from build123d import *

# Parameters (mm, degrees)
SKETCH1_R           = 1.7
BOSS_EXTRUDE1_DEPTH = 13.5
CUT_EXTRUDE2_START  = -3.5
CUT_EXTRUDE2_DEPTH  = 3.5
BOSS_EXTRUDE2_DEPTH = 15.5
CHAMFER1_SIZE       = 3


with BuildPart() as part:
    # Sketch1 → Boss-Extrude1 (new body)
    with BuildSketch(Plane(origin=(0, 3, 0), x_dir=(1, 0, 0), z_dir=(0, 1, 0))):
        with BuildLine():
            Line((71.5, -48.5), (71.5, 48.5))
            ThreePointArc((71.5, 48.5), (70.621320344, 50.621320344), (68.5, 51.5))
            Line((68.5, 51.5), (-68.5, 51.5))
            ThreePointArc((-68.5, 51.5), (-70.621320344, 50.621320344), (-71.5, 48.5))
            Line((-71.5, 48.5), (-71.5, -48.5))
            ThreePointArc((-71.5, -48.5), (-70.621320344, -50.621320344), (-68.5, -51.5))
            Line((-68.5, -51.5), (68.5, -51.5))
            ThreePointArc((68.5, -51.5), (70.621320344, -50.621320344), (71.5, -48.5))
        make_face()
        with Locations(Location((-64, 44, 0), (0, 0, 90))):
            Circle(SKETCH1_R, mode=Mode.SUBTRACT)
        with Locations(Location((-64, -44, 0), (0, 0, 90))):
            Circle(SKETCH1_R, mode=Mode.SUBTRACT)
        with Locations(Location((64, -44, 0), (0, 0, 90))):
            Circle(SKETCH1_R, mode=Mode.SUBTRACT)
        with Locations(Location((64, 44, 0), (0, 0, 90))):
            Circle(SKETCH1_R, mode=Mode.SUBTRACT)
    extrude(amount=-BOSS_EXTRUDE1_DEPTH)

    # Sketch2 → Cut-Extrude2 (cut)
    with BuildSketch(Plane.XZ.offset(10.5).offset(CUT_EXTRUDE2_START)):
        with BuildLine():
            Line((-71.5, -40.5), (-63, -40.5))
            Line((-63, -40.5), (-60.5, -43))
            Line((-60.5, -43), (-60.5, -51.5))
            Line((-60.5, -51.5), (-68.5, -51.5))
            ThreePointArc((-68.5, -51.5), (-70.621320344, -50.621320344), (-71.5, -48.5))
            Line((-71.5, -48.5), (-71.5, -40.5))
        make_face()
        with BuildLine():
            Line((-71.5, 40.5), (-63, 40.5))
            Line((-63, 40.5), (-60.5, 43))
            Line((-60.5, 43), (-60.5, 51.5))
            Line((-60.5, 51.5), (-68.5, 51.5))
            ThreePointArc((-68.5, 51.5), (-70.621320344, 50.621320344), (-71.5, 48.5))
            Line((-71.5, 48.5), (-71.5, 40.5))
        make_face()
        with BuildLine():
            Line((60.5, 51.5), (60.5, 43))
            Line((60.5, 43), (63, 40.5))
            Line((63, 40.5), (71.5, 40.5))
            Line((71.5, 40.5), (71.5, 48.5))
            ThreePointArc((71.5, 48.5), (70.621320344, 50.621320344), (68.5, 51.5))
            Line((68.5, 51.5), (60.5, 51.5))
        make_face()
        with BuildLine():
            Line((60.5, -51.5), (60.5, -43))
            Line((60.5, -43), (63, -40.5))
            Line((63, -40.5), (71.5, -40.5))
            Line((71.5, -40.5), (71.5, -48.5))
            ThreePointArc((71.5, -48.5), (70.621320344, -50.621320344), (68.5, -51.5))
            Line((68.5, -51.5), (60.5, -51.5))
        make_face()
    extrude(amount=CUT_EXTRUDE2_DEPTH, mode=Mode.SUBTRACT)

    # Sketch3 → Boss-Extrude2 (add)
    with BuildSketch(Plane.XZ.offset(10.5)):
        Polygon((-52.5, 46), (-52.5, -32), (-47, -37.5), (43, -37.5), (48.5, -32), (48.5, 46), (43, 51.5), (-47, 51.5), align=None)
    extrude(amount=BOSS_EXTRUDE2_DEPTH)

    # Chamfer1
    chamfer1_edges = [part.edges().sort_by_distance(p)[0] for p in [
        (-2, -26, -37.5),
        (-49.75, -26, -34.75),
        (48.5, -26, 7),
        (45.75, -26, -34.75),
        (45.75, -26, 48.75),
        (-2, -26, 51.5),
        (-49.75, -26, 48.75),
        (-52.5, -26, 7),
    ]]
    chamfer(chamfer1_edges, length=CHAMFER1_SIZE)


solid = part.part
The listing builds one solid part. Answer for the finished solid, in the listing's coordinates (mm). A direction names the side the tool comes from. Coordinates: 2 decimals unless noted, no trailing zeros. Write each loop counter-clockwise with the first axis right and the second up, starting at its lowest first coordinate (ties: lowest second). Pieces come first, ordered by that corner, then holes. Notation, with made-up numbers: M -22.5,-18 L 33.5,-18 A12 ccw 33.5,4 Z; hole C -14.75,61.5 d10. An arc over 180 degrees is marked long. Use one line per item in the form item = value.
Item 1: For faces 1 (the face through (-3, -17, -37.5)), 2 (the face through (-66, -7, -46)), 3 (the face through (66, -7, -46)), 4 (the face through (-67, -9, 40.5)), determine the directions among +Z, -Z, +X, -X, +Y, -Y from which every point of the face is accessible in a straight line to the end or side of a thin tool.
Model answer:
face_1 = -Z, +X, -X, -Y
face_2 = -Z, -X, -Y
face_3 = -Z, +X, -Y
face_4 = +Z, -X, -Y
Item 2: Find section B-B, the plane y = -19. Give the vertices of the cut face in (x, z).
Model answer:
outline = M -52.5,-32 L -47,-37.5 L 43,-37.5 L 48.5,-32 L 48.5,46 L 43,51.5 L -47,51.5 L -52.5,46 Z
Item 3: Find section C-C, the plane z = 20.5. Give the vertices of the cut face in (x, y), plus the area to 3 significant figures.
Model answer:
outline = M -71.5,-10.5 L -52.5,-10.5 L -52.5,-23 L -49.5,-26 L 45.5,-26 L 48.5,-23 L 48.5,-10.5 L 71.5,-10.5 L 71.5,3 L -71.5,3 Z
area = 3,490 mm2
Item 4: The mould has two halves that part along X. Classify faces 5 (the face through (-65.15, -1.93, 45.25)), 6 (the face through (-67, -9, -40.5)), 7 (the face through (-60.5, -9, 47)): released by +X, released by -X, zero draft, split by the parting line, or undercut.
Model answer:
face_5 = undercut
face_6 = zero draft
face_7 = released by -X
Item 5: Find section A-A, the plane x = 33. Give the vertices of the cut face in (y, z), plus the area to 3 significant figures.
Model answer:
outline = M -26,-34.5 L -23,-37.5 L -10.5,-37.5 L -10.5,-51.5 L 3,-51.5 L 3,51.5 L -23,51.5 L -26,48.5 Z
area = 2,760 mm2
Item 6: Given P1, Ø1.8, axis at y = -8.5, z = 47, coming from the -X side; P2, Ø5.5, axis at x = -67.5, z = -46.5, coming from the -Y side; P3, Ø1.8, axis at y = -8.5, z = 48, coming from the +X side; P4, Ø4, axis at x = -64, z = -44, coming from the +Y side, each flat-ended and moving along its own axis, determine where each tip first touches the part or whether it passes through.
Model answer:
P1 = -60.5
P2 = -7
P3 = 60.5
P4 = 3
Item 7: Find the intervals of material crossed by probe 1 along X at (y, z) = (-0.75, -44); probe 2 along Y at (x, z) = (53.5, 4.5); probe 3 along Z at (x, y) = (-42, -22), in increasing order.
Model answer:
probe_1 = -71.5 to -65.7, -62.3 to 62.3, 65.7 to 71.5
probe_2 = -10.5 to 3
probe_3 = -37.5 to 51.5
Item 8: Find section D-D, the plane x = 53. Give the vertices of the cut face in (y, z).
Model answer:
outline = M -10.5,-51.5 L 3,-51.5 L 3,51.5 L -10.5,51.5 Z
